from build123d import *

# Parameters (mm, degrees)
F0_W      = 80
F0_H      = 10
F1_DEPTH  = 5
F3_DEPTH  = 5
F6_DEPTH  = 5
F9_DEPTH  = 5
F12_DEPTH = 5
F14_DEPTH = 5


with BuildPart() as f1:
    # F0 (on Top) → F1 (new body)
    with BuildSketch(Plane.XY):
        with Locations((40, 5)):
            Rectangle(F0_W, F0_H)
    extrude(amount=F1_DEPTH)

    # F2 (on Right) → F3 (join)
    with BuildSketch(Plane.YZ):
        Polygon((-4.9618040211, 0), (0, 0), (0, 2.0297223236), (-4.097959958, 2.0297223236), (-5.8396296574, 4.6212524176), (-5.8396296574, 6.2223259127), (-4.17390365, 7.4121300131), (-5.360500887, 9.073366411), (-7.6862322167, 7.4121300131), (-7.6862322167, 5.0199492835), align=None)
    extrude(amount=F3_DEPTH)

    # F5 (on offset) → F6 (join)
    with BuildSketch(Plane.YZ.offset(20)):
        Polygon((-4.9618040211, 0), (0, 0), (0, 2.0297223236), (-4.097959958, 2.0297223236), (-5.8396296574, 4.6212524176), (-5.8396296574, 6.2223259127), (-4.17390365, 7.4121300131), (-5.360500887, 9.073366411), (-7.6862322167, 7.4121300131), (-7.6862322167, 5.0199492835), align=None)
    extrude(amount=F6_DEPTH)

    # F8 (on offset) → F9 (join)
    with BuildSketch(Plane.YZ.offset(50)):
        Polygon((-5.360500887, 9.073366411), (-7.6862322167, 7.4121300131), (-7.6862322167, 5.0199492835), (-4.9618040211, 0), (0, 0), (0, 2.0297223236), (-4.097959958, 2.0297223236), (-5.8396296574, 4.6212524176), (-5.8396296574, 6.2223259127), (-4.17390365, 7.4121300131), align=None)
    extrude(amount=F9_DEPTH)

    # F11 (on offset) → F12 (join)
    with BuildSketch(Plane.YZ.offset(75)):
        Polygon((-5.8396296574, 6.2223259127), (-4.17390365, 7.4121300131), (-5.360500887, 9.073366411), (-7.6862322167, 7.4121300131), (-7.6862322167, 5.0199492835), (-4.9618040211, 0), (0, 0), (0, 2.0297223236), (-4.097959958, 2.0297223236), (-5.8396296574, 4.6212524176), align=None)
    extrude(amount=F12_DEPTH)

    # F13 (on face) → F14 (join)
    with BuildSketch(Plane.XY.offset(5)):
        Polygon((8.3886766806, 30.3718596697), (0, 13.1700793281), (25.1010470092, 13.2027473301), (25.1010470092, 10), (54.7285676003, 10), (54.7285676003, 13.4966513142), (71.5840160847, 13.4966513142), (80, 30.7553019375), (54.801363498, 30.7553019375), (54.801363498, 36.3780027509), (25.2450443804, 36.3780027509), (25.2450443804, 30.3718596697), align=None)
        Polygon((30.0217233598, 17.5636745989), (7.3759490624, 17.5260230899), (11.2720150501, 25.5676303059), (30.0217233598, 25.5676303059), (30.0217233598, 31.4697995782), (49.8536489904, 31.4697995782), (49.8536489904, 26.3000894338), (72.4333301187, 26.3000894338), (68.5819346344, 18.350683593), (49.8536489904, 18.350683593), (49.8536489904, 12.2224157676), (30.0217233598, 12.2224157676), align=None, mode=Mode.SUBTRACT)
    extrude(amount=-F14_DEPTH)


solid = f1.part
Work out the finished part from the listing and answer in its coordinate system (mm). A direction names the side the tool comes from. Coordinates: 2 decimals unless noted, no trailing zeros. Loops run counter-clockwise (first coordinate to the right, second up) from the corner with the lowest first, then second, coordinate; pieces in that order, holes last. Notation, with made-up numbers: M 54,23 L 74,23 A17 cw 74,28 Z; hole C 66,-29.75 d5. An arc over 180 degrees is marked long. Answer in a Markdown table with one row per item. Add a question column.
1. Find section C-C, the plane x = 33. Write down the section's boundary in (y, z), then the cut area to 3 significant figures.
2. Consider L1, parallel to X at y = -6, z = 2; L2, parallel to Y at x = 23, z = 0.5; L3, parallel to Y at x = 39, z = 4. Determine where each line is inside the solid, lowest interval first.
3. Flat-ended cylindrical pins translate along their axes: P1, Ø1.5, axis at x = 10, z = 1.5, coming from the +Y side; P2, Ø1.5, axis at x = 72, z = 2, coming from the +Y side; P3, Ø6, axis at x = 38.5, y = 27, coming from the +Z side; P4, Ø1.5, axis at x = 11, z = 5.5, coming from the -Y side. Find the tip coordinate at first contact, or state that the pin passes through.
4. Find section A-A, the plane x = 51.5. Write down the section's boundary in (y, z).
5. The mould has two halves that part along X. Classify faces 1 (the flat face through (0, 1, 3)), 2 (the flat face through (75, -5, 3)), 3 (the flat face through (39, 11, 0)): pulls with the +X half, pulls with the -X half, needs draft (parallel to the pull), parting line crosses it, or undercut.
6. Find section D-D, the plane x = 10.5. Write down the section's boundary in (y, z).
7. A tool of negligible diameter and unlimited length cuts with its end or side. For faces 4 (the flat face through (70.535, 22.381, 2.535)), 5 (the flat face through (2.46, -5.02, 6.81)), 6 (the flat face through (52, -5.84, 5)), 7 (the flat face through (67, 10, 2)), from which of +Z, -Z, +X, -X, +Y, -Y can it reach the whole face along a straight path? Write none if from no direction.
8. Find section B-B, the plane y = -1. Write down the section's boundary in (x, z).
Reported:
| question | item | result |
|---|---|---|
| 1 | outline | M 0,0 L 12.22,0 L 12.22,5 L 0,5 Z; M 31.47,0 L 36.38,0 L 36.38,5 L 31.47,5 Z |
| 1 | area | 85.7 mm^2 |
| 2 | L1 | x = 0 to 5, 20 to 25, 50 to 55, 75 to 80 |
| 2 | L2 | y = -5.23 to 10, 13.2 to 17.55, 25.57 to 30.37 |
| 2 | L3 | y = 0 to 12.22, 31.47 to 36.38 |
| 3 | P1 | stops at y = 30.37 |
| 3 | P2 | stops at y = 30.76 |
| 3 | P3 | passes through |
| 3 | P4 | stops at y = 0 |
| 4 | outline | M -7.69,5.02 L -4.96,0 L 18.35,0 L 18.35,5 L 0,5 L 0,2.03 L -4.1,2.03 L -5.84,4.62 L -5.84,6.22 L -4.17,7.41 L -5.36,9.07 L -7.69,7.41 Z; M 26.3,0 L 36.38,0 L 36.38,5 L 26.3,5 Z |
| 5 | face 1 | pulls with the -X half |
| 5 | face 2 | undercut |
| 5 | face 3 | needs draft |
| 6 | outline | M 0,0 L 10,0 L 10,5 L 0,5 Z; M 13.18,0 L 17.53,0 L 17.53,5 L 13.18,5 Z; M 23.97,0 L 30.37,0 L 30.37,5 L 23.97,5 Z |
| 7 | face 4 | +Z, -Z |
| 7 | face 5 | +X, -X, +Y |
| 7 | face 6 | +X, -X |
| 7 | face 7 | +Z, -Z, +X |
| 8 | outline | M 0,0 L 5,0 L 5,2.03 L 0,2.03 Z; M 20,0 L 25,0 L 25,2.03 L 20,2.03 Z; M 50,0 L 55,0 L 55,2.03 L 50,2.03 Z; M 75,0 L 80,0 L 80,2.03 L 75,2.03 Z |
